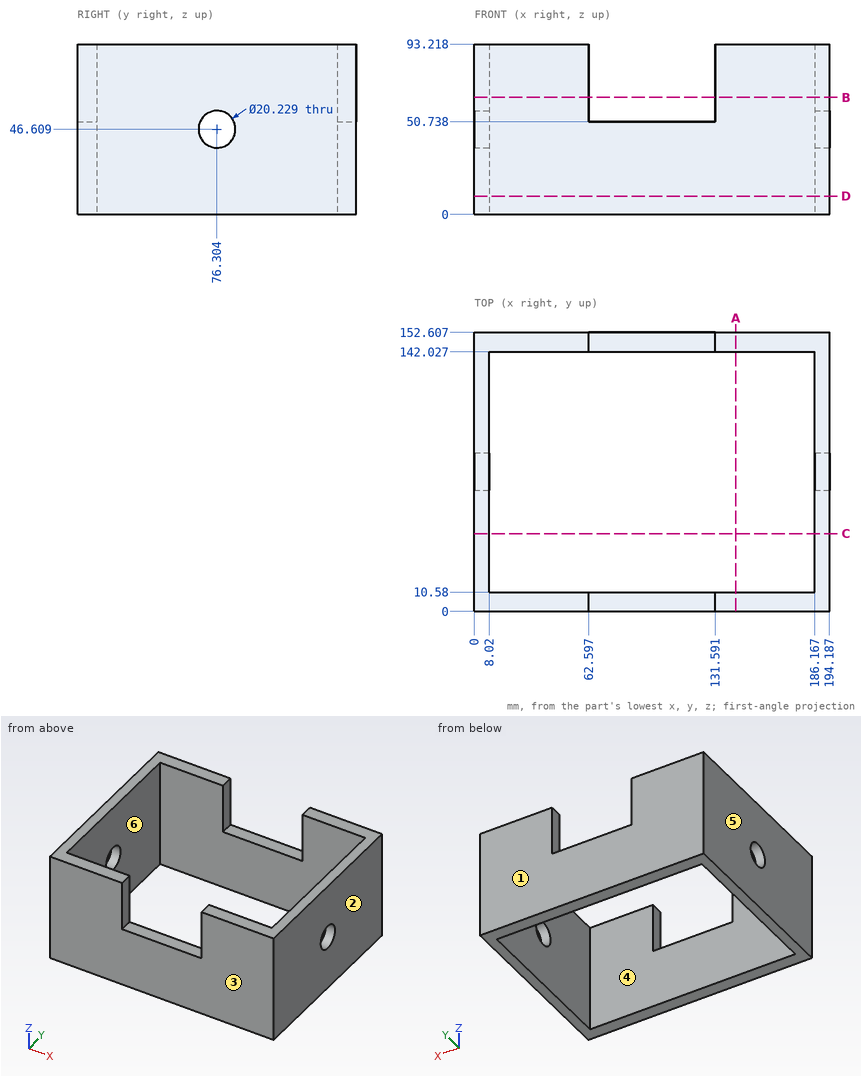
Geometry check sheet. Reference: drawing and pictorial views, mm from the part's lowest x, y, z. A direction names the side the tool comes from. Give positions to 0.01 mm unless a question says otherwise; leave off trailing zeros. Loops run counter-clockwise (first coordinate to the right, second up) from the corner with the lowest first, then second, coordinate; pieces in that order, holes last. Notation, with made-up numbers: M 23.5,63 L 66.5,63 A15 ccw 66.5,85 Z; hole C -3,63.5 d8. An arc over 180 degrees is marked long. Use a Markdown table: item, result. Add a question column.
Q1. Go/stop test with flat-tipped pins: pin 1 (18 mm diameter, centred on y = 76.3, z = 46.61, fed in from -X); pin 2 (3 mm diameter, centred on x = 105.5, y = 3, fed in from +Z). Record where each tip stops, or that it passes through.
Q2. Sectioned sample at D-D, the plane z = 10. Record the cut outline in (x, y), then the cut area to 3 significant figures.
Q3. Sectioned sample at A-A, the plane x = 143. Record the cut outline in (y, z), then the cut area to 3 significant figures.
Q4. Sectioned sample at B-B, the plane z = 64. Record the cut outline in (x, y), then the cut area to 3 significant figures.
Q5. Scan lines: line 1 along Y through (x, z) = (28.5, 60); line 2 along X through (y, z) = (91.5, 14). Record each from-to range of solid material in increasing order. Write a range as [from, to].
Q6. Tool access check on the marked faces 5 and 6. Record the directions out of +Z, -Z, +X, -X, +Y, -Y that give a thin tool (end or side, any length) a straight path to the whole face; none if there is none.
Q7. Mould release check, pull along Y, two halves, no side actions. Record for the marked faces 1, 2, 3 and 4: pulls with the +Y half, pulls with the -Y half, needs draft (parallel to the pull), parting line crosses it, or undercut.
Q8. Sectioned sample at C-C, the plane y = 42.5. Record the cut outline in (x, z).
Verdict:
| question | item | result |
|---|---|---|
| 1 | pin 1 | through |
| 1 | pin 2 | z = 50.74 |
| 2 | outline | M 0,0 L 194.19,0 L 194.19,152.61 L 0,152.61 Z; hole M 8.02,10.58 L 186.17,10.58 L 186.17,142.03 L 8.02,142.03 Z |
| 2 | area | 6,220 mm^2 |
| 3 | outline | M 0,0 L 10.58,0 L 10.58,93.22 L 0,93.22 Z; M 142.03,0 L 152.61,0 L 152.61,93.22 L 142.03,93.22 Z |
| 3 | area | 1,970 mm^2 |
| 4 | outline | M 0,0 L 62.6,0 L 62.6,10.58 L 8.02,10.58 L 8.02,142.03 L 62.6,142.03 L 62.6,152.61 L 0,152.61 Z; M 131.59,0 L 194.19,0 L 194.19,152.61 L 131.59,152.61 L 131.59,142.03 L 186.17,142.03 L 186.17,10.58 L 131.59,10.58 Z |
| 4 | area | 4,760 mm^2 |
| 5 | line 1 | [0, 10.58], [142.03, 152.61] |
| 5 | line 2 | [0, 8.02], [186.17, 194.19] |
| 6 | face 5 | +Z, -Z, -X, +Y, -Y |
| 6 | face 6 | +Z, -Z |
| 7 | face 1 | pulls with the +Y half |
| 7 | face 2 | needs draft |
| 7 | face 3 | pulls with the -Y half |
| 7 | face 4 | undercut |
| 8 | outline | M 0,0 L 8.02,0 L 8.02,93.22 L 0,93.22 Z; M 186.17,0 L 194.19,0 L 194.19,93.22 L 186.17,93.22 Z |
